Read the model definition and answer for the solid it produces. Units are mm, in the model's axes. A direction names the side the tool comes from. Coordinates: 2 decimals unless noted, no trailing zeros. Order: outer loops, then holes, each group sorted by start corner. A loop starts at its lowest first (then second) coordinate and runs counter-clockwise, first axis right, second up. Notation, with made-up numbers: (-23, 47) -> (6, 47) arc R10 cw to (6, 64) -> close; hole circle Ø11 at (47, 76.25). An arc over 180 degrees is marked (long way). Return JSON: item names as keys, results as strings. Group by question number.
```python
from build123d import *

# Parameters (mm, degrees)
SKETCH1_R      = 6.35
EXTRUDE1_DEPTH = 9.525


with BuildPart() as part:
    # Sketch1 → Extrude1 (new body)
    with BuildSketch(Plane.XY):
        with BuildLine():
            Line((0, 0), (139.7, 0))
            Line((139.7, 0), (139.7, 26.173786324))
            ThreePointArc((139.7, 26.173786324), (140.092825695, 30.022467519), (141.255102041, 33.712423164))
            ThreePointArc((141.255102041, 33.712423164), (130.016323799, 83.311919995), (79.358899418, 87.811428571))
            ThreePointArc((79.358899418, 87.811428571), (74.63797582, 85.782960673), (69.546649161, 85.09))
            Line((69.546649161, 85.09), (0, 85.09))
            Line((0, 85.09), (0, 0))
        make_face()
        with Locations(Location((101.6, 50.8, 0), (0, 0, 180))):
            Circle(SKETCH1_R, mode=Mode.SUBTRACT)
    extrude(amount=EXTRUDE1_DEPTH)


solid = part.part
```
1. Which of the six approach directions +Z, -Z, +X, -X, +Y, -Y give full straight-line access (tool end or side, diameter ignored) to faces 4 (the face through (35, 85.09, 5)), 5 (the face through (0, 43, 5)), 6 (the face through (139.7, 13, 5))?
2. Straight lines are drawn through the part: L1, parallel to X at y = 50.8, z = 3; L2, parallel to Y at x = 101.6, z = 6; L3, parallel to X at y = 6.5, z = 6.5. For each, find the intervals that lie inside material, in ascending order.
3. Find section A-A on y = 50.8. Determine the outline of the cut face in (x, z) (3 decimals), and give its area (3 significant figures).
4. For a pull along Y with two mould halves and no side action, classify faces 1 (the face through (71, 48, 9.525)), 2 (the face through (107.944, 50.521, 4.696)), 3 (the face through (140.082, 29.969, 4.696)) as released by +Y, released by -Y, zero draft, split by the parting line, or undercut.
5. Given pin 1 (1 mm diameter, centred on y = 71, z = 1.5, fed in from -X), flat-ended and moving along its own axis, determine where the tip first touches the part or whether it passes through.
6. Find section D-D on y = 21. Determine the outline of the cut face in (x, z) (3 decimals).
7. Find section C-C on x = 101.6. Determine the outline of the cut face in (y, z) (3 decimals), and give its area (3 significant figures).
8. Find section B-B on z = 4.75. Determine the outline of the cut face in (x, y), and give its area (3 significant figures).
Result:
{
 "1": {"face 4": "+Z, -Z, -X, +Y", "face 5": "+Z, -Z, -X, +Y, -Y", "face 6": "+Z, -Z, +X, -Y"},
 "2": {"L1": "0 to 95.25, 107.95 to 144.78", "L2": "0 to 44.45, 57.15 to 93.98", "L3": "0 to 139.7"},
 "3": {"outline": "(0, 0) -> (95.25, 0) -> (95.25, 9.525) -> (0, 9.525) -> close; (107.95, 0) -> (144.78, 0) -> (144.78, 9.525) -> (107.95, 9.525) -> close", "area": "1,260 mm^2"},
 "4": {"face 1": "zero draft", "face 2": "undercut", "face 3": "released by -Y"},
 "5": {"pin 1": "x = 0"},
 "6": {"outline": "(0, 0) -> (139.7, 0) -> (139.7, 9.525) -> (0, 9.525) -> close"},
 "7": {"outline": "(0, 0) -> (44.45, 0) -> (44.45, 9.525) -> (0, 9.525) -> close; (57.15, 0) -> (93.98, 0) -> (93.98, 9.525) -> (57.15, 9.525) -> close", "area": "774 mm^2"},
 "8": {"outline": "(0, 0) -> (139.7, 0) -> (139.7, 26.17) arc R19.05 cw to (141.26, 33.71) arc R43.18 ccw to (79.36, 87.81) arc R19.05 cw to (69.55, 85.09) -> (0, 85.09) -> close; hole circle Ø12.7 at (101.6, 50.8)", "area": "12,200 mm^2"}
}
